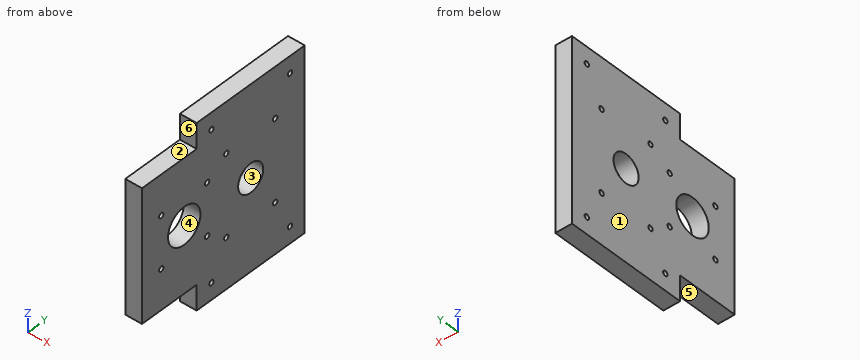
```python
from build123d import *

# Parameters (mm, degrees)
SKETCH_1_R      = 1.5
SKETCH_1_R_2    = 8.5
SKETCH_1_R_3    = 11
EXTRUDE_1_DEPTH = 10


with BuildPart() as part:
    # 草图1 → 凸台-拉伸1 (new body)
    with BuildSketch(Plane(origin=(0, 0, 0), x_dir=(0, 0, -1), z_dir=(1, 0, 0))):
        Polygon((-27.5, 36.58), (-47.5, 36.58), (-47.5, -36.58), (-32.5, -36.58), (-32.5, -73.58), (46.13, -73.58), (46.13, -36.58), (61.13, -36.58), (61.13, 36.58), align=None)
        with Locations((-8.685, -29.5)):
            Circle(SKETCH_1_R, mode=Mode.SUBTRACT)
        with Locations((-37.5, 26.58)):
            Circle(SKETCH_1_R, mode=Mode.SUBTRACT)
        with Locations((-17.5, 16.58)):
            Circle(SKETCH_1_R, mode=Mode.SUBTRACT)
        with Locations((31.13, 16.58)):
            Circle(SKETCH_1_R, mode=Mode.SUBTRACT)
        with Locations((51.13, 26.58)):
            Circle(SKETCH_1_R, mode=Mode.SUBTRACT)
        with Locations((-37.5, -26.58)):
            Circle(SKETCH_1_R, mode=Mode.SUBTRACT)
        with Locations((-17.5, -16.58)):
            Circle(SKETCH_1_R, mode=Mode.SUBTRACT)
        with Locations((31.13, -16.58)):
            Circle(SKETCH_1_R, mode=Mode.SUBTRACT)
        with Locations((51.13, -26.58)):
            Circle(SKETCH_1_R, mode=Mode.SUBTRACT)
        with Locations((22.315, -29.5)):
            Circle(SKETCH_1_R, mode=Mode.SUBTRACT)
        with Locations((-8.685, -60.5)):
            Circle(SKETCH_1_R, mode=Mode.SUBTRACT)
        with Locations((22.315, -60.5)):
            Circle(SKETCH_1_R, mode=Mode.SUBTRACT)
        with Locations((6.815, 0)):
            Circle(SKETCH_1_R_2, mode=Mode.SUBTRACT)
        with Locations((6.815, -45)):
            Circle(SKETCH_1_R_3, mode=Mode.SUBTRACT)
    extrude(amount=EXTRUDE_1_DEPTH)


solid = part.part
```
Check sheet for the modelled part. Datum: model origin and axes. Units: mm. Face numbers are marked on the shaded views. A direction names the side the tool comes from. Give positions to 0.01 mm unless a question says otherwise; leave off trailing zeros. Loops run counter-clockwise (first coordinate to the right, second up) from the corner with the lowest first, then second, coordinate; pieces in that order, holes last. Notation, with made-up numbers: M 40,-32.75 L 68,-32.75 A13 cw 68,-24.75 Z; hole C 42.5,-16.5 d11. An arc over 180 degrees is marked long. Answer in a Markdown table with one row per item.
1) Cross-section at A-A (y = -45). Enter the section's corners in (x, z) (3 decimals).
Solutions:
| item | result |
|---|---|
| outline | M 0,-46.13 L 10,-46.13 L 10,-17.815 L 0,-17.815 Z; M 0,4.185 L 10,4.185 L 10,32.5 L 0,32.5 Z |
2) Tool access check on the marked faces 1 and 2. Record the directions out of +Z, -Z, +X, -X, +Y, -Y that give a thin tool (end or side, any length) a straight path to the whole face; none if there is none.
Solutions:
| item | result |
|---|---|
| face 1 | +Z, -Z, -X, +Y, -Y |
| face 2 | +Z, +X, -X, -Y |
3) Cross-section at B-B (z = -51.13). Enter the section's corners in (x, y), plus the area to 3 significant figures.
Solutions:
| item | result |
|---|---|
| outline | M 0,-36.58 L 10,-36.58 L 10,-28.08 L 0,-28.08 Z; M 0,-25.08 L 10,-25.08 L 10,25.08 L 0,25.08 Z; M 0,28.08 L 10,28.08 L 10,36.58 L 0,36.58 Z |
| area | 672 mm^2 |
4) Thickness scan on line 1 (Y direction, x = 2.5, z = 37.5); line 2 (Y direction, x = 5.5, z = -31.13); line 3 (Z direction, x = 2.5, y = -29). Record the ranges inside material, lowest first.
Solutions:
| item | result |
|---|---|
| line 1 | y = -36.58 to -28.08, -25.08 to 25.08, 28.08 to 36.58 |
| line 2 | y = -73.58 to -18.08, -15.08 to 15.08, 18.08 to 36.58 |
| line 3 | z = -61.13 to -23.73, -20.9 to 7.27, 10.1 to 47.5 |
5) Cross-section at D-D (x = 4.75). Count the separate pieces of the cut face and the enclosed holes in it, plus the area to 3 significant figures.
Solutions:
| item | result |
|---|---|
| separate pieces | 1 |
| enclosed holes | 14 |
| area | 10,200 mm^2 |
6) Depth check by flat-ended pin: pin 1 (6 mm diameter, centred on y = -29.5, z = 11.5, fed in from -X); pin 2 (2.5 mm diameter, centred on y = 16.58, z = 17.5, fed in from -X); pin 3 (6 mm diameter, centred on x = 4, y = -45.5, fed in from +Z); pin 4 (5 mm diameter, centred on x = 3.5, z = 41.5, fed in from -Y). Enter the tip coordinate at first touch or a pass-through.
Solutions:
| item | result |
|---|---|
| pin 1 | stops at x = 0 |
| pin 2 | passes through |
| pin 3 | stops at z = 32.5 |
| pin 4 | stops at y = -36.58 |
7) Cross-section at C-C (y = -60.5). Enter the section's corners in (x, z) (3 decimals).
Solutions:
| item | result |
|---|---|
| outline | M 0,-46.13 L 10,-46.13 L 10,-23.815 L 0,-23.815 Z; M 0,-20.815 L 10,-20.815 L 10,7.185 L 0,7.185 Z; M 0,10.185 L 10,10.185 L 10,32.5 L 0,32.5 Z |
8) Mould release check, pull along Z, two halves, no side actions. Record for the marked faces 3, 4, 5 and 6: released by +Z, released by -Z, zero draft, split by the parting line, or undercut.
Solutions:
| item | result |
|---|---|
| face 3 | undercut |
| face 4 | undercut |
| face 5 | released by -Z |
| face 6 | zero draft |
